Here's how the part is built. I have some questions about the finished solid (model axes, mm). A direction names the side the tool comes from. Give positions to 0.01 mm unless a question says otherwise; leave off trailing zeros. Order: outer loops, then holes, each group sorted by start corner. A loop starts at its lowest first (then second) coordinate and runs counter-clockwise, first axis right, second up.
Autodesk Inventor part; units mm, degrees
ref_plane "YZ Plane" through (0, 0, 0) normal (1, 0, 0) x (0, 1, 0)
ref_plane "XZ Plane" through (0, 0, 0) normal (0, 1, 0) x (-1, 0, 0)
ref_plane "XY Plane" through (0, 0, 0) normal (0, 0, 1) x (1, 0, 0)
sketch "Sketch1" plane through (0, 0, 0) normal (0, 0, 1) x (1, 0, 0)
  line L0 (0, 0) -> (0, -18.18) construction
  line L1 (0, -18.18) -> (-15, -18.18) construction
  line L2 (-15, -18.18) -> (-15, -16.18)
  line L3 (-15, -16.18) -> (-9, -16.18) construction
  line L4 (-9, -16.18) -> (0, 0) construction
  line L5 (-10.1443, -16.18) -> (-6.6868, -9.9643)
  line L6 (-5.4267, -11.8132) -> (-8.9682, -18.18)
  line L7 (-15, -16.18) -> (-10.1443, -16.18)
  line L8 (-15, -18.18) -> (-8.9682, -18.18)
  line L9 (15, -18.18) -> (15, -16.18)
  line L10 (15, -16.18) -> (9, -16.18) construction
  line L11 (10.1443, -16.18) -> (6.6868, -9.9643)
  line L12 (5.4267, -11.8132) -> (8.9682, -18.18)
  line L13 (15, -16.18) -> (10.1443, -16.18)
  line L14 (15, -18.18) -> (8.9682, -18.18)
  arc A0 (-5.4267, -11.8132) -> (5.4267, -11.8132) centre (0, 0) ccw
  arc A1 (6.6868, -9.9643) -> (-6.6868, -9.9643) centre (0, 0) ccw
  dimension "d1" = 15
  dimension "d2" = 18.18
  dimension "d3" = 2
  dimension "d4" = 6
  dimension "d5" = 1
  dimension "d6" = 2
  dimension "d9" = 12
  dimension "d10" = 13
extrude "Extrusion1" add sketch "Sketch1" along normal mid plane 20
sketch "Sketch2" plane through (0, 0, 0) normal (0, 0, 1) x (1, 0, 0)
  arc A0 (6.6868, -9.9643) -> (-6.6868, -9.9643) centre (0, 0) ccw
  circle A1 centre (0, 0) radius 12
extrude "Extrusion2" add sketch "Sketch2" along normal mid plane 25
chamfer "Chamfer1" distance 2 angle 45 2 edges at (-12, 0, 12.5) (-12, 0, -12.5)
properties part number "Motor"
Q1. If we section it at B-B on y = 0: List the corners of the cut face in (x, z) for me.
Filled sheet:
outline: (-12, -10.5) - (-10, -12.5) - (10, -12.5) - (12, -10.5) - (12, 10.5) - (10, 12.5) - (-10, 12.5) - (-12, 10.5) - close
Q2. If we section it at C-C on x = 0: List the corners of the cut face in (y, z) for me.
Filled sheet:
outline: (-13, -10) - (-12, -10) - (-12, -10.5) - (-10, -12.5) - (10, -12.5) - (12, -10.5) - (12, 10.5) - (10, 12.5) - (-10, 12.5) - (-12, 10.5) - (-12, 10) - (-13, 10) - close
Q3. I need wall thicknesses on L1, parallel to X at y = -12, z = 0.5; L2, parallel to Y at x = -13.25, z = -2.5; L3, parallel to Z at x = -12, y = -17. Which ranges of each line are inside material? Lowest first, please.
Filled sheet:
L1: x = -7.82 to -5.53, -5 to 5, 5.53 to 7.82
L2: y = -18.18 to -16.18
L3: z = -10 to 10
Q4. Thinking about a two-plate mould opening in Y: for faces 1 (the face through (13, -16.18, 0)), 2 (the face through (8.44, -13.12, -0.14)), 3 (the face through (-12, -18.18, 0)), 4 (the face through (1, -12.5, -10)), which applies, released by +Y, released by -Y, zero draft, split by the parting line, or undercut?
Filled sheet:
face 1: undercut
face 2: undercut
face 3: released by -Y
face 4: zero draft
Q5. I'm going to push flat-ended pins straight in: P1, Ø5.5, axis at x = 13, z = 1, coming from the +Y side; P2, Ø10, axis at x = 2.5, z = 4.5, coming from the -Y side; P3, Ø8, axis at y = -11, z = -8.5, coming from the +X side. Where does each tip first touch, or does it pass through?
Filled sheet:
P1: stops at y = 6.24
P2: stops at y = -15.54
P3: stops at x = 9.75
Q6. For faces 5 (the face through (0.1, -12, 10.2)), 6 (the face through (0.1, -12, -10.3)), 7 (the face through (-8.44, -13.12, -0.14)), 8 (the face through (-7.2, -15, -0.1)), which set-ups out of +Z, -Z, +X, -X, +Y, -Y let a thin tool reach every point of the face, with its end or its side?
Filled sheet:
face 5: +Z, -Y
face 6: -Z, -Y
face 7: +Z, -Z, -X
face 8: +Z, -Z, -Y
Q7. If we section it at A-A on z = -8.25: List the corners of the cut face in (x, y) for me, plus the area to 3 significant figures.
Filled sheet:
outline: (-15, -18.18) - (-8.97, -18.18) - (-5.43, -11.81) arc R13 ccw to (5.43, -11.81) - (8.97, -18.18) - (15, -18.18) - (15, -16.18) - (10.14, -16.18) - (6.69, -9.96) arc R12 ccw (long way) to (-6.69, -9.96) - (-10.14, -16.18) - (-15, -16.18) - close
area: 516 mm2
